Geometry check sheet. Reference: the model listing, model coordinates, mm. Face numbers are marked on the shaded views. A direction names the side the tool comes from. Round coordinates to 2 decimals unless told otherwise and drop trailing zeros. Order: outer loops, then holes, each group sorted by start corner. A loop starts at its lowest first (then second) coordinate and runs counter-clockwise, first axis right, second up. Notation, with made-up numbers: M -22.75,67.5 L 21.25,67.5 A15 cw 21.25,79.5 Z; hole C 45.5,13 d8. An arc over 180 degrees is marked long. Answer as a JSON object with one key per item and string values. Group by question number.
Solid Edge part; units mm, degrees
sketch "Sketch1" plane through (0, 0, -203.2) normal (0, 0, 1) x (1, 0, 0)
  line L0 (-101.6, -95.25) -> (-101.6, 95.25)
  line L1 (-101.6, 95.25) -> (-99.695, 95.25)
  line L2 (-99.695, 95.25) -> (-99.695, 107.95)
  line L3 (-99.695, 107.95) -> (-85.725, 107.95)
  line L4 (-85.725, -107.95) -> (-99.695, -107.95)
  line L5 (-99.695, -107.95) -> (-99.695, -95.25)
  line L6 (-99.695, -95.25) -> (-101.6, -95.25)
  dimension "D1" = 99.695
revolve "RevolvedProtrusion1" add sketch "Sketch1" angle 360 about axis through (-85.725, 107.95, -203.2) along (0, -1, 0)
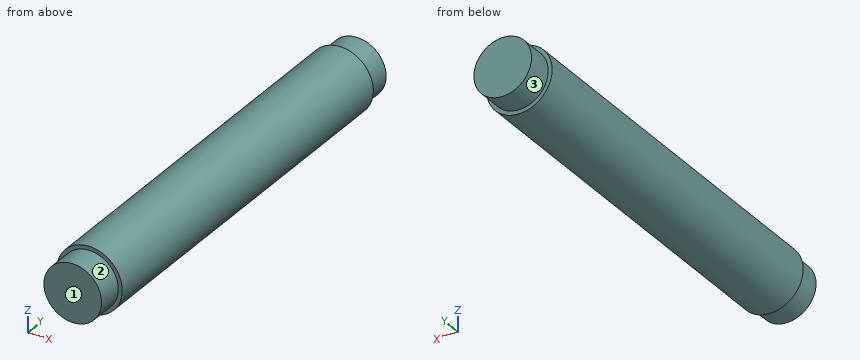
1) Go/stop test with flat-tipped pins: P1, Ø3, axis at x = -96.5, y = -18.5, coming from the +Z side; P2, Ø12, axis at y = -6, z = -213.5, coming from the -X side; P3, Ø1.5, axis at y = -82.5, z = -205.5, coming from the +X side. Record where each tip stops, or that it passes through.
2) Sectioned sample at B-B (x = -74.5). Record the boundary of the cut face in (y, z), then the cut area to 3 significant figures.
3) Sectioned sample at C-C (y = -65). Record the boundary of the cut face in (x, z) (3 decimals), then the cut area to 3 significant figures.
4) Thickness scan on line 1 along Y through (x, z) = (-71.5, -207.5); line 2 along Z through (x, y) = (-73.5, 58); line 3 along X through (y, z) = (9, -213). Record the ranges inside material, lowest first. Write a range as [from, to].
5) Set-up check for the marked faces 1, 2 and 3: record each of +Z, -Z, +X, -X, +Y, -Y from which the full face is reachable in a straight line by a thin tool's end or side.
6) Sectioned sample at A-A (z = -191.5). Record the boundary of the cut face in (x, y), then the cut area to 3 significant figures.
Final values:
{
 "1": {"P1": "stops at z = -190.32", "P2": "stops at x = -101.01", "P3": "stops at x = -69.93"},
 "2": {"outline": "M -107.95,-211.52 L -95.25,-211.52 L -95.25,-214.43 L 95.25,-214.43 L 95.25,-211.52 L 107.95,-211.52 L 107.95,-194.88 L 95.25,-194.88 L 95.25,-191.97 L -95.25,-191.97 L -95.25,-194.88 L -107.95,-194.88 Z", "area": "4,700 mm^2"},
 "3": {"outline": "C -85.725,-203.2 d31.75", "area": "792 mm^2"},
 "4": {"line 1": "y = [-95.25, 95.25]", "line 2": "z = [-213.33, -193.07]", "line 3": "x = [-98.21, -73.24]"},
 "5": {"face 1": "+Z, -Z, +X, -X, -Y", "face 2": "-Y", "face 3": "+Y"},
 "6": {"outline": "M -96.45,-95.25 L -93.36,-95.25 L -93.36,-107.95 L -78.09,-107.95 L -78.09,-95.25 L -75,-95.25 L -75,95.25 L -78.09,95.25 L -78.09,107.95 L -93.36,107.95 L -93.36,95.25 L -96.45,95.25 Z", "area": "4,480 mm^2"}
}
